```python
from build123d import *

# Parameters (mm, degrees)
EXTRUDE1_DEPTH     = 0.635
SKETCH2_R          = 1.5875
EXTRUDE2_DEPTH     = 1.635
SKETCH3_R          = 1.1303
EXTRUDE3_DEPTH     = 1.016
EXTRUDE4_DEPTH     = 0.635
SKETCH5_R          = 1.1303
CUT_EXTRUDE1_DEPTH = 2.016


with BuildPart() as part:
    # Sketch1 → Extrude1 (new body)
    with BuildSketch(Plane(origin=(0, 0, 0), x_dir=(0, 0, -1), z_dir=(1, 0, 0))):
        Polygon((16.178476913, 44.45), (0, 0), (-101.6, 21.595746666), (-101.6, 31.120746666), (-73.015323979, 44.45), align=None)
    extrude(amount=EXTRUDE1_DEPTH)

    # Sketch2 → Extrude2 (cut, through all)
    with BuildSketch(Plane.ZY):
        with Locations((8.531149291, 4.410096871)):
            Circle(SKETCH2_R)
        with Locations((33.37609835, 9.691053818)):
            Circle(SKETCH2_R)
        with Locations((58.221047409, 14.972010765)):
            Circle(SKETCH2_R)
        with Locations((83.065996467, 20.252967712)):
            Circle(SKETCH2_R)
    extrude(amount=-EXTRUDE2_DEPTH, mode=Mode.SUBTRACT)

    # Sketch4 → Extrude4 (cut)
    with BuildSketch(Plane.ZY):
        Polygon((73.015323979, 44.45), (-16.178476913, 44.45), (0, 0), (101.6, 21.595746666), (101.6, 31.120746666), align=None)
    extrude(amount=-EXTRUDE4_DEPTH, mode=Mode.SUBTRACT)


with BuildPart() as body_2:
    # Sketch3 → Extrude3 (new body)
    with BuildSketch(Plane.ZY.offset(-0.635)):
        Polygon((-16.178476913, 44.45), (0, 0), (101.6, 21.595746666), (101.6, 31.120746666), (73.015323979, 44.45), align=None)
        with Locations((8.531149291, 4.410096871)):
            Circle(SKETCH3_R, mode=Mode.SUBTRACT)
        with Locations((33.37609835, 9.691053818)):
            Circle(SKETCH3_R, mode=Mode.SUBTRACT)
        with Locations((58.221047409, 14.972010765)):
            Circle(SKETCH3_R, mode=Mode.SUBTRACT)
        with Locations((83.065996467, 20.252967712)):
            Circle(SKETCH3_R, mode=Mode.SUBTRACT)
        Polygon((7.516900107, 39.6875), (-9.376922031, 39.6875), (3.059330207, 5.519177793), (18.74002683, 8.852212752), align=None, mode=Mode.SUBTRACT)
        Polygon((23.444235817, 9.852123239), (39.124932441, 13.185158198), (29.478868887, 39.6875), (12.585046748, 39.6875), align=None, mode=Mode.SUBTRACT)
        Polygon((34.547015528, 39.6875), (43.829141428, 14.185068686), (59.509838051, 17.518103645), (51.440837666, 39.6875), align=None, mode=Mode.SUBTRACT)
        Polygon((56.508984307, 39.6875), (64.214047038, 18.518014132), (96.8375, 25.452343124), (96.8375, 28.086699549), (71.959503148, 39.6875), align=None, mode=Mode.SUBTRACT)
    extrude(amount=-EXTRUDE3_DEPTH)

    # Sketch5 → Cut-Extrude1 (cut, through all)
    with BuildSketch(Plane(origin=(1.651, 0, 0), x_dir=(0, 0, -1), z_dir=(1, 0, 0))):
        with Locations((-11.55326057, 35.56)):
            Circle(SKETCH5_R)
    extrude(amount=-CUT_EXTRUDE1_DEPTH, mode=Mode.SUBTRACT)


solid = body_2.part
```
The model under review builds one solid part; all positions refer to its coordinate system, in mm. A direction names the side the tool comes from. Coordinates: 2 decimals unless noted, no trailing zeros. Write each loop counter-clockwise with the first axis right and the second up, starting at its lowest first coordinate (ties: lowest second). Pieces come first, ordered by that corner, then holes. Notation, with made-up numbers: (1, 60.5) -> (54, 60.5) arc R26 ccw to (54, 79.5) -> close; hole circle Ø4 at (6, 89). An arc over 180 degrees is marked (long way). One line per item, written item: value. Start each with the question number.
Q1. Clearance check with flat-ended pins moving along their axes: P1, Ø0.5, axis at x = 1, y = 26, coming from the -Z side; P2, Ø5, axis at y = 18, z = 53.5, coming from the +X side; P3, Ø1.4, axis at y = 35.56, z = 11.55, coming from the -X side; P4, Ø0.5, axis at x = 1, z = 61.5, coming from the -Y side. State where each tip first meets the part, or that it passes through.
Q2. The part is to be moulded in two halves that separate along Z. For faces 3 (the face through (1.136, 10.647, 50.089)), 4 (the face through (1.1, 11.5, 31.2)), 5 (the face through (1.651, 29, 38)), say which applies: +Z half, -Z half, draft (parallel to the pull), parting line (faces both ways), or undercut.
Q3. To check wall thickness, follow probe 1 along Z at (x, y) = (0.9, 27); probe 2 along Z at (x, y) = (0.75, 35); probe 3 along Z at (x, y) = (1.35, 32.5). State the ranges of each line that lie inside material, in increasing order.
Q4. For faces 1 (the face through (1.14, 26.25, 34.37)), 2 (the face through (1.136, 22.536, -8.202)), list the 3-axis set-ups (+Z, -Z, +X, -X, +Y, -Y) from which the entire face can be reached by the end or side of a thin tool; tool diameter is ignored.
Q5. Add section C-C, the plane x = 1.1. Count the separate pieces of the cut face and the enclosed holes in it, then the cut area to 3 significant figures.
Q6. Add section A-A, the plane y = 23. Give the boundary of the cut face in (x, z) (3 decimals).
Q7. Add section B-B, the plane z = 77. Give the boundary of the cut face in (x, y) (3 decimals).
Q8. Add section D-D, the plane y = 35.56. Give the boundary of the cut face in (x, z) (3 decimals).
Response:
1. P1: z = -9.55
1. P2: x = 1.65
1. P3: through
1. P4: y = 13.02
2. face 3: +Z half
2. face 4: undercut
2. face 5: draft
3. probe 1: -9.83 to -4.76, 12.13 to 17.2, 34.1 to 39.16, 56.06 to 61.13, 96.84 to 101.6
3. probe 2: -12.74 to -7.67, 9.22 to 10.57, 12.54 to 14.29, 31.18 to 36.25, 53.15 to 58.22, 82.01 to 93.28
3. probe 3: -11.83 to -6.76, 10.13 to 15.2, 32.09 to 37.16, 54.06 to 59.13, 87.37 to 98.64
4. face 1: +X, -X
4. face 2: -Z, +X, -X, -Y
5. separate pieces: 1
5. enclosed holes: 9
5. area: 1,630 mm²
6. outline: (0.635, -8.371) -> (1.651, -8.371) -> (1.651, -3.303) -> (0.635, -3.303) -> close; (0.635, 13.591) -> (1.651, 13.591) -> (1.651, 18.659) -> (0.635, 18.659) -> close; (0.635, 35.553) -> (1.651, 35.553) -> (1.651, 40.621) -> (0.635, 40.621) -> close; (0.635, 57.515) -> (1.651, 57.515) -> (1.651, 62.583) -> (0.635, 62.583) -> close; (0.635, 85.3) -> (1.651, 85.3) -> (1.651, 101.6) -> (0.635, 101.6) -> close
7. outline: (0.635, 16.367) -> (1.651, 16.367) -> (1.651, 21.236) -> (0.635, 21.236) -> close; (0.635, 37.337) -> (1.651, 37.337) -> (1.651, 42.592) -> (0.635, 42.592) -> close
8. outline: (0.635, -12.943) -> (1.651, -12.943) -> (1.651, -7.875) -> (0.635, -7.875) -> close; (0.635, 9.019) -> (1.651, 9.019) -> (1.651, 10.423) -> (0.635, 10.423) -> close; (0.635, 12.684) -> (1.651, 12.684) -> (1.651, 14.087) -> (0.635, 14.087) -> close; (0.635, 30.981) -> (1.651, 30.981) -> (1.651, 36.049) -> (0.635, 36.049) -> close; (0.635, 52.943) -> (1.651, 52.943) -> (1.651, 58.011) -> (0.635, 58.011) -> close; (0.635, 80.811) -> (1.651, 80.811) -> (1.651, 92.08) -> (0.635, 92.08) -> close
